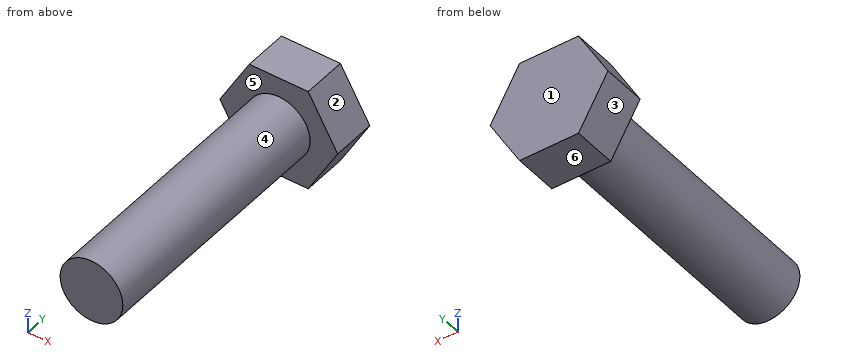
from build123d import *

# Parameters (mm, degrees)
BOSS_EXTRUDE1_DEPTH = 5.5
BOSS_EXTRUDE2_START = -32
SKETCH2_R           = 3.9
BOSS_EXTRUDE2_DEPTH = 32


with BuildPart() as part:
    # Sketch1 → Boss-Extrude1 (new body)
    with BuildSketch(Plane(origin=(0, 0, 0), x_dir=(1, 0, 0), z_dir=(0, 1, 0))):
        Polygon((7.332348419, 0), (3.666174209, 6.35), (-3.666174209, 6.35), (-7.332348419, 0), (-3.666174209, -6.35), (3.666174209, -6.35), align=None)
    extrude(amount=BOSS_EXTRUDE1_DEPTH)

    # Sketch2 → Boss-Extrude2 (add)
    with BuildSketch(Plane(origin=(0, 0, 0), x_dir=(1, 0, 0), z_dir=(0, 1, 0)).offset(BOSS_EXTRUDE2_START)):
        with Locations(Location((0, 0, 0), (0, 0, 270))):
            Circle(SKETCH2_R)
    extrude(amount=BOSS_EXTRUDE2_DEPTH)


solid = part.part
Here's how the part is built. I have some questions about the finished solid (model axes, mm). Face numbers are marked on the shaded views. A direction names the side the tool comes from. Give positions to 0.01 mm unless a question says otherwise; leave off trailing zeros. Order: outer loops, then holes, each group sorted by start corner. A loop starts at its lowest first (then second) coordinate and runs counter-clockwise, first axis right, second up. Notation, with made-up numbers: (60, 72) -> (67, 72) arc R9 ccw to (67, 86) -> close; hole circle Ø8 at (5.5, 82). An arc over 180 degrees is marked (long way). Use a Markdown table: item, result. Add a question column.
Item 1: Imagine slicing it at A-A on x = 0. Please give me the cut outline in (y, z).
Item 2: Imagine slicing it at B-B on z = -1.75. Please give me the cut outline in (x, y).
Item 3: I need wall thicknesses on line 1 (Y direction, x = 3.75, z = -5.75); line 2 (X direction, y = -29.5, z = 1.25). Which ranges of each line are inside material? Lowest first, please.
Item 4: Will these pins go through, and if not, where does the flat tip stop? pin 1 (2 mm diameter, centred on x = 5.5, y = -4.5, fed in from -Z); pin 2 (6 mm diameter, centred on x = -5, y = -15.5, fed in from +Z).
Item 5: Imagine slicing it at D-D on y = -24.5. Please give me the cut outline in (x, z).
Item 6: If we mould it in two halves opening along X, with no side actions, what happens to the marked faces 1, 2, 3 and 4? For each: pulls with the +X half, pulls with the -X half, needs draft (parallel to the pull), parting line crosses it, or undercut.
Item 7: Imagine slicing it at C-C on y = 1. Please give me the cut outline in (x, z).
Item 8: For the marked faces 5 and 6, which set-ups out of +Z, -Z, +X, -X, +Y, -Y let a thin tool reach every point of the face, with its end or its side?
Data:
| question | item | result |
|---|---|---|
| 1 | outline | (-32, -3.9) -> (0, -3.9) -> (0, -6.35) -> (5.5, -6.35) -> (5.5, 6.35) -> (0, 6.35) -> (0, 3.9) -> (-32, 3.9) -> close |
| 2 | outline | (-6.32, 0) -> (-3.49, 0) -> (-3.49, -32) -> (3.49, -32) -> (3.49, 0) -> (6.32, 0) -> (6.32, 5.5) -> (-6.32, 5.5) -> close |
| 3 | line 1 | y = 0 to 5.5 |
| 3 | line 2 | x = -3.69 to 3.69 |
| 4 | pin 1 | passes through |
| 4 | pin 2 | stops at z = 3.35 |
| 5 | outline | circle Ø7.8 at (0, 0) |
| 6 | face 1 | needs draft |
| 6 | face 2 | pulls with the +X half |
| 6 | face 3 | pulls with the -X half |
| 6 | face 4 | parting line crosses it |
| 7 | outline | (-7.33, 0) -> (-3.67, -6.35) -> (3.67, -6.35) -> (7.33, 0) -> (3.67, 6.35) -> (-3.67, 6.35) -> close |
| 8 | face 5 | -Y |
| 8 | face 6 | -Z, +X, -X, +Y, -Y |
